CAD build for the part. Positions are in the model's coordinates, mm. Face numbers are marked on the shaded views. A direction names the side the tool comes from. Coordinates: 2 decimals unless noted, no trailing zeros. Write each loop counter-clockwise with the first axis right and the second up, starting at its lowest first coordinate (ties: lowest second). Pieces come first, ordered by that corner, then holes. Notation, with made-up numbers: (11.25, 8.25) -> (65.25, 8.25) arc R17 cw to (65.25, 40.25) -> close; hole circle Ø11 at (-8, -13.5). An arc over 180 degrees is marked (long way). Answer as CSV lines item,"result". Start each with the question number.
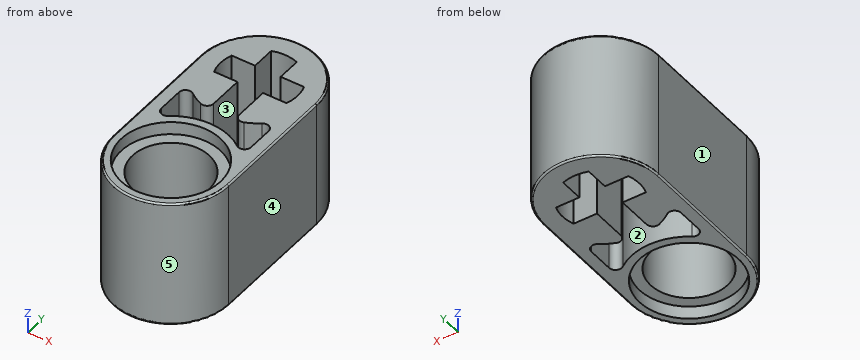
Autodesk Inventor part; units mm, degrees
ref_plane "YZ Plane" through (0, 0, 0) normal (1, 0, 0) x (0, 1, 0)
ref_plane "XZ Plane" through (0, 0, 0) normal (0, 1, 0) x (-1, 0, 0)
ref_plane "XY Plane" through (0, 0, 0) normal (0, 0, 1) x (1, 0, 0)
sketch "Sketch1" plane through (0, 0, 0) normal (0, 0, 1) x (1, 0, 0)
  line L0 (3.6, 0) -> (3.6, 8)
  line L1 (-3.6, 8) -> (-3.6, 0)
  arc A0 (3.6, 8) -> (-3.6, 8) centre (0, 8) ccw
  circle A1 centre (0, 8) radius 2.4 construction
  circle A2 centre (0, 8) radius 3.2 construction
  circle A3 centre (0, 0) radius 3.2
  circle A4 centre (0, 0) radius 2.4
  line L2 (0, 0) -> (0, 8) construction
  line L3 (-2.8, 5.7373) -> (-2.8, 2.2627)
  line L4 (2.8, 5.7373) -> (2.8, 2.2627)
  arc A5 (-2.8, 5.7373) -> (2.8, 5.7373) centre (0, 8) ccw
  arc A6 (2.8, 2.2627) -> (-2.8, 2.2627) centre (0, 0) ccw
  arc A7 (-3.6, 0) -> (3.6, 0) centre (0, 0) ccw
  line L5 (0.8, 4.49) -> (0.8, 7.2)
  line L6 (0.8, 7.2) -> (2.2627, 7.2)
  line L7 (2.2627, 8.8) -> (0.8, 8.8)
  line L8 (0.8, 8.8) -> (0.8, 10.2627)
  line L9 (-0.8, 10.2627) -> (-0.8, 8.8)
  line L10 (-0.8, 8.8) -> (-2.2627, 8.8)
  line L11 (-2.2627, 7.2) -> (-0.8, 7.2)
  line L12 (-0.8, 7.2) -> (-0.8, 4.49)
  arc A8 (-2.2627, 8.8) -> (-2.2627, 7.2) centre (0, 8) ccw
  arc A9 (0.8, 10.2627) -> (-0.8, 10.2627) centre (0, 8) ccw
  arc A10 (2.2627, 7.2) -> (2.2627, 8.8) centre (0, 8) ccw
  dimension "d8" = 4.8
  dimension "d9" = 6.4
  dimension "d32" = 7.2
  dimension "d34" = 8
  dimension "d36" = 0.8
  dimension "d52" = 1.6
extrude "Extrusion1" add sketch "Sketch1" along normal mid plane 8 contours A7 L1 A0 L0 | A3
sketch "Sketch6" plane through (0, 0, 4) normal (0, 0, 1) x (1, 0, 0)
  circle A0 centre (0, 0) radius 3.1
  circle A1 centre (0, 0) radius 2.4
  dimension "d53" = 6.2
extrude "Extrusion7" cut sketch "Sketch6" against normal blind 0.8 contours A0 | A1
mirror "Mirror1" about plane through (0, 0, 0) normal (0, 0, 1) of "Extrusion7"
fillet "Fillet1" radius 0.1 6 edges at (0, 11.6, 4) (3.6, 4, 4) (-3.6, 4, 4) (0, 11.6, -4) (-3.6, 4, -4) (3.6, 4, -4)
fillet "Fillet1" radius 0.4 6 edges at (-2.8, 5.7373, 0) (-2.8, 2.2627, 0) (2.8, 2.2627, 0) (2.8, 5.7373, 0) (0.8, 4.49, 0) (-0.8, 4.49, 0)
equation "\"d8\" = kd"
equation "\"d9\" = tsd"
equation "\"d32\" = tlad"
equation "\"d34\" = lu"
equation "\"d52\" = axlet"
equation "\"d14\" = lu"
equation "\"d41\" = tsl"
equation "\"d45\" = lf"
equation "\"d46\" = tf"
properties part number "60483-Black" material "ABS Plastic"
1. Wall check: line 1 (Y direction, x = 0, z = 1); line 2 (Y direction, x = 0, z = -3.7); line 3 (Y direction, x = 1.75, z = 2.5). Give the ranges that are in metal, low to high.
2. Cut at A-A (z = -0.25). Give the cut face in (x, y), then the cut area to 3 significant figures.
3. Mould opens along Y. For the marked faces 3, 4 and 5 say: pulls with the +Y half, pulls with the -Y half, needs draft (parallel to the pull), parting line crosses it, or undercut.
4. Flat gauge pins, fed straight in: P1, Ø2, axis at x = 3, z = 1.5, coming from the +Y side; P2, Ø1.6, axis at y = 9.5, z = 2, coming from the +X side; P3, Ø0.7, axis at x = -1.5, z = -1.5, coming from the +Y side. Where does each tip first touch, or does it go through?
5. Tool access for the marked faces 1 and 2: list every direction of +Z, -Z, +X, -X, +Y, -Y with a clear straight run to the whole face (end or side of a thin tool).
6. Cut at C-C (y = 7.5). Give the cut face in (x, z), then the cut area to 3 significant figures.
7. Cut at B-B (x = 0). Give the cut face in (y, z).
8. Cut at D-D (z = 3.5). Give the cut face in (x, y), then the cut area to 3 significant figures.
Geometry check:
1,line 1,"-3.6 to -2.4, 2.4 to 3.6, 10.4 to 11.6"
1,line 2,"-3.6 to -3.1, 3.1 to 3.6, 10.4 to 11.6"
1,line 3,"-3.15 to -1.64, 1.64 to 3.15, 4.85 to 7.2, 8.8 to 11.15"
2,outline,"(-3.6, 0) arc R3.6 ccw to (3.6, 0) -> (3.6, 8) arc R3.6 ccw to (-3.6, 8) -> close; hole (-2.8, 3.2) arc R0.4 ccw to (-2.16, 2.88) arc R3.6 cw to (2.16, 2.88) arc R0.4 ccw to (2.8, 3.2) -> (2.8, 4.8) arc R0.4 ccw to (2.16, 5.12) arc R3.6 cw to (1.35, 4.66) arc R0.4 cw to (0.8, 5.03) -> (0.8, 7.2) -> (2.26, 7.2) arc R2.4 ccw to (2.26, 8.8) -> (0.8, 8.8) -> (0.8, 10.26) arc R2.4 ccw to (-0.8, 10.26) -> (-0.8, 8.8) -> (-2.26, 8.8) arc R2.4 ccw to (-2.26, 7.2) -> (-0.8, 7.2) -> (-0.8, 5.03) arc R0.4 cw to (-1.35, 4.66) arc R3.6 cw to (-2.16, 5.12) arc R0.4 ccw to (-2.8, 4.8) -> close; hole circle Ø4.8 at (0, 0)"
2,area,"57.3 mm²"
3,face 3,"undercut"
3,face 4,"needs draft"
3,face 5,"pulls with the -Y half"
4,P1,"y = 10.99"
4,P2,"x = 3.53"
4,P3,"y = 11.41"
5,face 1,"+Z, -Z, -X, +Y, -Y"
5,face 2,"+Z, -Z"
6,outline,"(-3.6, -3.9) arc R0.1 ccw to (-3.5, -4) -> (-2.35, -4) -> (-2.35, 4) -> (-3.5, 4) arc R0.1 ccw to (-3.6, 3.9) -> close; (2.35, -4) -> (3.5, -4) arc R0.1 ccw to (3.6, -3.9) -> (3.6, 3.9) arc R0.1 ccw to (3.5, 4) -> (2.35, 4) -> close"
6,area,"20.0 mm²"
7,outline,"(-3.6, -3.9) arc R0.1 ccw to (-3.5, -4) -> (-3.1, -4) -> (-3.1, -3.2) -> (-2.4, -3.2) -> (-2.4, 3.2) -> (-3.1, 3.2) -> (-3.1, 4) -> (-3.5, 4) arc R0.1 ccw to (-3.6, 3.9) -> close; (2.4, -3.2) -> (3.1, -3.2) -> (3.1, -4) -> (3.6, -4) -> (3.6, 4) -> (3.1, 4) -> (3.1, 3.2) -> (2.4, 3.2) -> close; (10.4, -4) -> (11.5, -4) arc R0.1 ccw to (11.6, -3.9) -> (11.6, 3.9) arc R0.1 ccw to (11.5, 4) -> (10.4, 4) -> close"
8,outline,"(-3.6, 0) arc R3.6 ccw to (3.6, 0) -> (3.6, 8) arc R3.6 ccw to (-3.6, 8) -> close; hole circle Ø6.2 at (0, 0); hole (-2.8, 3.2) arc R0.4 ccw to (-2.16, 2.88) arc R3.6 cw to (2.16, 2.88) arc R0.4 ccw to (2.8, 3.2) -> (2.8, 4.8) arc R0.4 ccw to (2.16, 5.12) arc R3.6 cw to (1.35, 4.66) arc R0.4 cw to (0.8, 5.03) -> (0.8, 7.2) -> (2.26, 7.2) arc R2.4 ccw to (2.26, 8.8) -> (0.8, 8.8) -> (0.8, 10.26) arc R2.4 ccw to (-0.8, 10.26) -> (-0.8, 8.8) -> (-2.26, 8.8) arc R2.4 ccw to (-2.26, 7.2) -> (-0.8, 7.2) -> (-0.8, 5.03) arc R0.4 cw to (-1.35, 4.66) arc R3.6 cw to (-2.16, 5.12) arc R0.4 ccw to (-2.8, 4.8) -> close"
8,area,"45.2 mm²"
